```python
from build123d import *

# Parameters (mm, degrees)
SKETCH_W        = 27.5
SKETCH_H        = 57.5
SKETCH_R        = 1.75
PAD_DEPTH       = 9
POCKET_DEPTH    = 7
SKETCH002_W     = 23.2
SKETCH002_H     = 54.5
POCKET001_DEPTH = 3
SKETCH003_W     = 0.8
SKETCH003_H     = 5
PAD001_DEPTH    = 1.4
CHAMFER_SIZE    = 0.6
SKETCH004_W     = 20
SKETCH004_H     = 3
POCKET002_DEPTH = 9.001
SKETCH005_W     = 21.5
SKETCH005_H     = 2
PAD002_DEPTH    = 2
POCKET003_DEPTH = 3
CHAMFER001_SIZE = 2.5


with BuildPart() as part:
    # Sketch → Pad (new body)
    with BuildSketch(Plane.XY):
        Rectangle(SKETCH_W, SKETCH_H)
        with Locations((-4.5, 9.25)):
            Circle(SKETCH_R, mode=Mode.SUBTRACT)
        with Locations((-4.5, -25.75)):
            Circle(SKETCH_R, mode=Mode.SUBTRACT)
        with Locations((4.5, 9.25)):
            Circle(SKETCH_R, mode=Mode.SUBTRACT)
        with Locations((4.5, -25.75)):
            Circle(SKETCH_R, mode=Mode.SUBTRACT)
    extrude(amount=PAD_DEPTH)

    # Sketch001 (on Face10 of Pad) → Pocket (cut)
    with BuildSketch(Plane.XY.offset(9)):
        Polygon((-10.5, 26), (10.5, 26), (10.5, -26), (8, -26), (8, -29), (-8, -29), (-8, -26), (-10.5, -26), align=None)
    extrude(amount=-POCKET_DEPTH, mode=Mode.SUBTRACT)

    # Sketch002 (on Face5 of Pocket) → Pocket001 (cut)
    with BuildSketch(Plane.XY.offset(9)):
        Rectangle(SKETCH002_W, SKETCH002_H)
    extrude(amount=-POCKET001_DEPTH, mode=Mode.SUBTRACT)

    # Sketch003 (on Face5 of Pocket001) → Pad001 (join)
    with BuildSketch(Plane.XY.offset(9)):
        with Locations((-11.2, 12.5)):
            Rectangle(SKETCH003_W, SKETCH003_H)
        with Locations((-11.2, -12.5)):
            Rectangle(SKETCH003_W, SKETCH003_H)
        with Locations((11.2, -12.5)):
            Rectangle(SKETCH003_W, SKETCH003_H)
        with Locations((11.2, 12.5)):
            Rectangle(SKETCH003_W, SKETCH003_H)
    extrude(amount=-PAD001_DEPTH)

    # Chamfer
    chamfer_edges = [part.edges().sort_by_distance(p)[0] for p in [
        (-10.8, -12.5, 9),
        (-10.8, -12.5, 7.6),
        (-10.8, 12.5, 9),
        (-10.8, 12.5, 7.6),
        (10.8, 12.5, 9),
        (10.8, 12.5, 7.6),
        (10.8, -12.5, 9),
        (10.8, -12.5, 7.6),
    ]]
    chamfer(chamfer_edges, length=CHAMFER_SIZE)

    # Sketch004 (on Face4 of Chamfer) → Pocket002 (cut, through all)
    with BuildSketch(Plane.XY.offset(9)):
        with Locations((0, 27.5)):
            Rectangle(SKETCH004_W, SKETCH004_H)
    extrude(amount=-POCKET002_DEPTH, mode=Mode.SUBTRACT)

    # Sketch005 (on Face22 of Pocket002) → Pad002 (join)
    with BuildSketch(Plane.XY.offset(2)):
        with Locations((0, 25.25)):
            Rectangle(SKETCH005_W, SKETCH005_H)
        with Locations((0, -20)):
            Rectangle(SKETCH005_W, SKETCH005_H)
    extrude(amount=PAD002_DEPTH)

    # Sketch006 (on Face54 of Pad002) → Pocket003 (cut)
    with BuildSketch(Plane.XY.offset(2)):
        with BuildLine():
            ThreePointArc((-7, 21.25), (-10.5, 17.75), (-7, 14.25))
            Line((-7, 14.25), (7, 14.25))
            ThreePointArc((7, 14.25), (10.5, 17.75), (7, 21.25))
            Line((-7, 21.25), (7, 21.25))
        make_face()
        with BuildLine():
            ThreePointArc((-1.5, 1), (-6, 5.5), (-10.5, 1))
            Line((-10.5, 1), (-10.5, -14))
            ThreePointArc((-10.5, -14), (-6, -18.5), (-1.5, -14))
            Line((-1.5, 1), (-1.5, -14))
        make_face()
        with BuildLine():
            ThreePointArc((10.5, 1), (6, 5.5), (1.5, 1))
            Line((1.5, 1), (1.5, -14))
            ThreePointArc((1.5, -14), (6, -18.5), (10.5, -14))
            Line((10.5, 1), (10.5, -14))
        make_face()
    extrude(amount=-POCKET003_DEPTH, mode=Mode.SUBTRACT)

    # Chamfer001
    chamfer001_edges = [part.edges().sort_by_distance(p)[0] for p in [
        (-13.75, 0, 0),
        (13.75, 0, 0),
    ]]
    chamfer(chamfer001_edges, length=CHAMFER001_SIZE)


solid = part.part
```
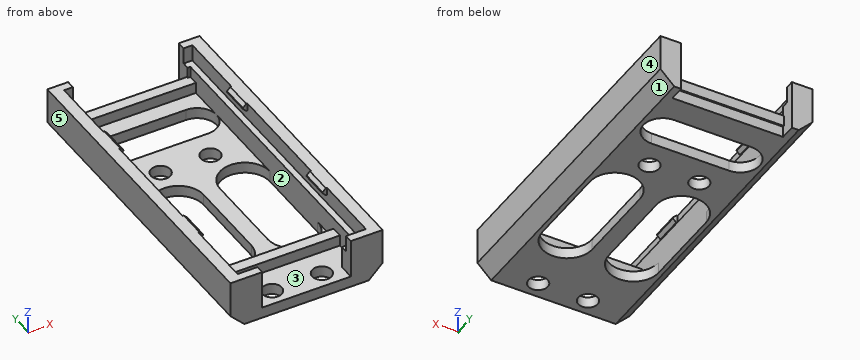
Work out the finished part from the listing and answer in its coordinate system (mm). Face numbers are marked on the shaded views. A direction names the side the tool comes from. Round coordinates to 2 decimals unless told otherwise and drop trailing zeros. Loops run counter-clockwise (first coordinate to the right, second up) from the corner with the lowest first, then second, coordinate; pieces in that order, holes last.
(1) The part is cut by section D-D, the plane y = 16. Give the vertices of the cut face in (x, z), and give its area (3 significant figures).
Computed values:
outline: (-13.75, 2.5) - (-11.25, 0) - (-10.03, 0) - (-10.03, 2) - (-10.5, 2) - (-10.5, 6) - (-11.6, 6) - (-11.6, 9) - (-13.75, 9) - close; (10.03, 0) - (11.25, 0) - (13.75, 2.5) - (13.75, 9) - (11.6, 9) - (11.6, 6) - (10.5, 6) - (10.5, 2) - (10.03, 2) - close
area: 47.5 mm2
(2) The part is cut by section B-B, the plane x = 0. Give the vertices of the cut face in (y, z).
Computed values:
outline: (-28.75, 0) - (14.25, 0) - (14.25, 2) - (-19, 2) - (-19, 4) - (-21, 4) - (-21, 2) - (-28.75, 2) - close; (21.25, 0) - (26, 0) - (26, 2) - (26.25, 2) - (26.25, 4) - (24.25, 4) - (24.25, 2) - (21.25, 2) - close
(3) Each of these flat-tipped pins is pushed along its axis until it touches: P1, Ø2, axis at x = 0.5, y = -9, coming from the +Z side; P2, Ø0.6, axis at x = 0, y = 25, coming from the +Z side; P3, Ø6, axis at x = -6.5, y = -10, coming from the +Z side; P4, Ø1.6, axis at x = -5, z = 3.5, coming from the +Y side. Where does it stop, or does it pass through?
Computed values:
P1: stops at z = 2
P2: stops at z = 4
P3: passes through
P4: stops at y = 26.25
(4) The mould has two halves that part along X. Classify the marked faces 3, 4 and 5: pulls with the +X half, pulls with the -X half, needs draft (parallel to the pull), parting line crosses it, or undercut.
Computed values:
face 3: undercut
face 4: pulls with the +X half
face 5: pulls with the -X half
(5) For the marked faces 1 and 2, determine the directions among +Z, -Z, +X, -X, +Y, -Y from which every point of the face is accessible in a straight line to the end or side of a thin tool.
Computed values:
face 1: -Z, +X, +Y, -Y
face 2: +Z
(6) Find the intervals of material crossed by L1, parallel to Y at x = 4.5, z = 0.75; L2, parallel to X at y = -20, z = 7.5; L3, parallel to X at y = 23.5, z = 4.5, in increasing order.
Computed values:
L1: y = -28.75 to -27.5, -24 to -18.24, 5.24 to 7.5, 11 to 14.25, 21.25 to 26
L2: x = -13.75 to -11.6, 11.6 to 13.75
L3: x = -13.75 to -10.5, 10.5 to 13.75
(7) The part is cut by section A-A, the plane y = 9.25. Give the vertices of the cut face in (x, z).
Computed values:
outline: (-13.75, 2.5) - (-11.25, 0) - (-6.25, 0) - (-6.25, 2) - (-10.5, 2) - (-10.5, 6) - (-11.6, 6) - (-11.6, 9) - (-13.75, 9) - close; (-2.75, 0) - (2.75, 0) - (2.75, 2) - (-2.75, 2) - close; (6.25, 0) - (11.25, 0) - (13.75, 2.5) - (13.75, 9) - (11.6, 9) - (11.6, 6) - (10.5, 6) - (10.5, 2) - (6.25, 2) - close
(8) The part is cut by section C-C, the plane x = 5. Give the vertices of the cut face in (y, z).
Computed values:
outline: (-28.75, 0) - (-27.43, 0) - (-27.43, 2) - (-28.75, 2) - close; (-24.07, 0) - (-18.39, 0) - (-18.39, 2) - (-19, 2) - (-19, 4) - (-21, 4) - (-21, 2) - (-24.07, 2) - close; (5.39, 0) - (7.57, 0) - (7.57, 2) - (5.39, 2) - close; (10.93, 0) - (14.25, 0) - (14.25, 2) - (10.93, 2) - close; (21.25, 0) - (26, 0) - (26, 2) - (26.25, 2) - (26.25, 4) - (24.25, 4) - (24.25, 2) - (21.25, 2) - close
